```python
from build123d import *

# Parameters (mm, degrees)
F0_W     = 105.6
F0_H     = 55
F0_R     = 1.6
F0_R_2   = 21
F0_R_3   = 12.5
F1_DEPTH = 7
F2_R     = 3.1
F2_R_2   = 1.6
F3_DEPTH = 1.5
F4_W     = 6
F4_H     = 2.5
F5_DEPTH = 7.001
F7_DEPTH = 4
F8_R     = 1.75
F9_DEPTH = 55.001


with BuildPart() as f1:
    # F0 (on Top) → F1 (new body)
    with BuildSketch(Plane.XY):
        with Locations((50.8, 26.65)):
            Rectangle(F0_W, F0_H)
        with Locations((14, 2.5)):
            Circle(F0_R, mode=Mode.SUBTRACT)
        with Locations((66.1, 7.6)):
            Circle(F0_R, mode=Mode.SUBTRACT)
        with Locations((96.52, 2.5)):
            Circle(F0_R, mode=Mode.SUBTRACT)
        with Locations((40, 26.65)):
            Circle(F0_R_2, mode=Mode.SUBTRACT)
        with Locations((15.3, 50.7)):
            Circle(F0_R, mode=Mode.SUBTRACT)
        with Locations((66.1, 35.5)):
            Circle(F0_R, mode=Mode.SUBTRACT)
        with Locations((85, 26.65)):
            Circle(F0_R_3, mode=Mode.SUBTRACT)
        with Locations((90.2, 50.7)):
            Circle(F0_R, mode=Mode.SUBTRACT)
    extrude(amount=F1_DEPTH)

    # F2 (on face) → F3 (join)
    with BuildSketch(Plane.XY.offset(7)):
        with Locations((15.3, 50.7)):
            Circle(F2_R)
        with Locations((15.3, 50.7)):
            Circle(F2_R_2, mode=Mode.SUBTRACT)
        with Locations((90.2, 50.7)):
            Circle(F2_R)
        with Locations((90.2, 50.7)):
            Circle(F2_R_2, mode=Mode.SUBTRACT)
        with Locations((66.1, 35.5)):
            Circle(F2_R)
        with Locations((66.1, 35.5)):
            Circle(F2_R_2, mode=Mode.SUBTRACT)
        with Locations((66.1, 7.6)):
            Circle(F2_R)
        with Locations((66.1, 7.6)):
            Circle(F2_R_2, mode=Mode.SUBTRACT)
        with Locations((96.52, 2.5)):
            Circle(F2_R)
        with Locations((96.52, 2.5)):
            Circle(F2_R_2, mode=Mode.SUBTRACT)
        with Locations((14, 2.5)):
            Circle(F2_R)
        with Locations((14, 2.5)):
            Circle(F2_R_2, mode=Mode.SUBTRACT)
    extrude(amount=F3_DEPTH)

    # F4 (on face) → F5 (cut, through all)
    with BuildSketch(Plane.XY.offset(7)):
        with Locations((75.8, 48.9)):
            Rectangle(F4_W, F4_H)
        with Locations((75.8, 4.4)):
            Rectangle(F4_W, F4_H)
        with Locations((25.8, 48.9)):
            Rectangle(F4_W, F4_H)
        with Locations((25.8, 4.4)):
            Rectangle(F4_W, F4_H)
    extrude(amount=-F5_DEPTH, mode=Mode.SUBTRACT)

    # F6 (on face) → F7 (cut)
    with BuildSketch(Plane(origin=(0, 0, 0), x_dir=(1, 0, 0), z_dir=(0, 0, -1))):
        Polygon((12.267949, -5.5), (15.732051, -5.5), (17.464102, -2.5), (15.732051, 0.5), (12.267949, 0.5), (10.535898, -2.5), align=None)
        Polygon((98.252051, 0.5), (94.787949, 0.5), (93.055898, -2.5), (94.787949, -5.5), (98.252051, -5.5), (99.984102, -2.5), align=None)
        Polygon((63.1, -5.867949), (63.1, -9.332051), (66.1, -11.064102), (69.1, -9.332051), (69.1, -5.867949), (66.1, -4.135898), align=None)
        Polygon((63.1, -33.767949), (63.1, -37.232051), (66.1, -38.964102), (69.1, -37.232051), (69.1, -33.767949), (66.1, -32.035898), align=None)
        Polygon((91.932051, -47.7), (88.467949, -47.7), (86.735898, -50.7), (88.467949, -53.7), (91.932051, -53.7), (93.664102, -50.7), align=None)
        Polygon((13.567949, -47.7), (11.835898, -50.7), (13.567949, -53.7), (17.032051, -53.7), (18.764102, -50.7), (17.032051, -47.7), align=None)
    extrude(amount=-F7_DEPTH, mode=Mode.SUBTRACT)

    # F8 (on face) → F9 (cut, through all)
    with BuildSketch(Plane(origin=(0, 54.15, 0), x_dir=(-1, 0, 0), z_dir=(0, 1, 0))):
        with Locations((-75.8, 3.5)):
            Circle(F8_R)
        with Locations((-25.8, 3.5)):
            Circle(F8_R)
    extrude(amount=-F9_DEPTH, mode=Mode.SUBTRACT)


solid = f1.part
```
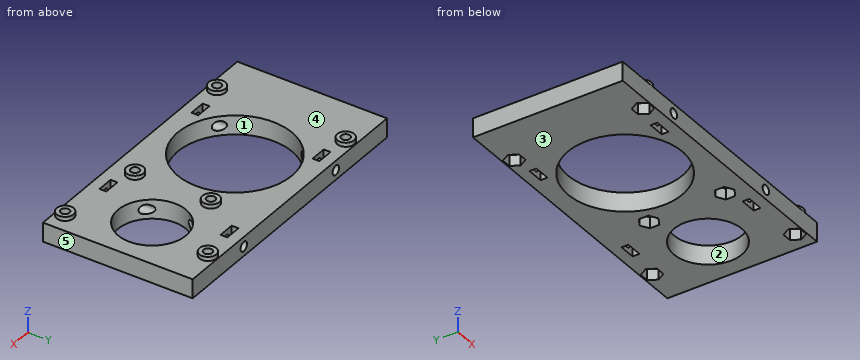
Could you check a few things on this model? Use its own coordinates, in mm. Face numbers are marked on the shaded views. A direction names the side the tool comes from. Round coordinates to 2 decimals unless told otherwise and drop trailing zeros. Order: outer loops, then holes, each group sorted by start corner. A loop starts at its lowest first (then second) coordinate and runs counter-clockwise, first axis right, second up. Notation, with made-up numbers: M -33,29.25 L 9,29.25 A17 ccw 9,52.25 Z; hole C -31.5,-36.75 d6. An arc over 180 degrees is marked long. One line per question, with ' | ' between items. Start each with the question number.
(1) Suppose I cut it at D-D on x = 90.2. List the corners of the cut face in (y, z) for me, then the cut area to 3 significant figures.
(2) Thinking about a two-plate mould opening in Y: for the marked faces 1, 2 and 3, which applies, +Y half, -Y half, draft (parallel to the pull), parting line (faces both ways), or undercut?
(3) Suppose I cut it at B-B on x = 40. List the corners of the cut face in (y, z) for me.
(4) Suppose I cut it at C-C on y = 7.6. List the corners of the cut face in (x, z) for me.
(5) Please list where these lines run through material, in increasing order: line 1 along X through (y, z) = (2.5, 6.7); line 2 along X through (y, z) = (50.7, 6.6); line 3 along Y through (x, z) = (40, 4.25).
(6) For P1, Ø5, axis at x = 76.5, z = 3, coming from the -Y side; P2, Ø4, axis at x = 44, y = 47.5, coming from the +Z side; P3, Ø1.9, axis at x = 90.2, y = 50.7, coming from the -Z side; P4, Ø5, axis at x = 15.3, y = 50.7, coming from the -Z side, each with a flat end and sliding along its axis, tell me the tip position at first contact or that it passes through.
(7) For the marked faces 4 and 5, which set-ups out of +Z, -Z, +X, -X, +Y, -Y let a thin tool reach every point of the face, with its end or its side?
(8) Suppose I cut it at A-A on y = 26.65. List the corners of the cut face in (x, z) for me, then the cut area to 3 significant figures.
Geometry results:
1) outline: M -0.85,0 L 15.28,0 L 15.28,7 L -0.85,7 Z; M 38.02,0 L 47.7,0 L 47.7,4 L 49.1,4 L 49.1,8.5 L 47.6,8.5 L 47.6,7 L 38.02,7 Z; M 52.3,4 L 53.7,4 L 53.7,0 L 54.15,0 L 54.15,7 L 53.8,7 L 53.8,8.5 L 52.3,8.5 Z | area: 197 mm²
2) face 1: undercut | face 2: undercut | face 3: draft
3) outline: M -0.85,0 L 5.65,0 L 5.65,7 L -0.85,7 Z; M 47.65,0 L 54.15,0 L 54.15,7 L 47.65,7 Z
4) outline: M -2,0 L 31.16,0 L 31.16,7 L -2,7 Z; M 48.84,0 L 63.1,0 L 63.1,4 L 64.5,4 L 64.5,8.5 L 63,8.5 L 63,7 L 48.84,7 Z; M 67.7,4 L 69.1,4 L 69.1,0 L 103.6,0 L 103.6,7 L 69.2,7 L 69.2,8.5 L 67.7,8.5 Z; hole C 25.8,3.5 d3.5; hole C 75.8,3.5 d3.5
5) line 1: -2 to 12.4, 15.6 to 94.92, 98.12 to 103.6 | line 2: -2 to 13.7, 16.9 to 88.6, 91.8 to 103.6 | line 3: -0.85 to 5.65, 47.65 to 54.15
6) P1: y = -0.85 | P2: z = 7 | P3: through | P4: z = 4
7) face 4: +Z | face 5: +Z, -Z, +X, +Y, -Y
8) outline: M -2,0 L 19,0 L 19,7 L -2,7 Z; M 61,0 L 72.5,0 L 72.5,7 L 61,7 Z; M 97.5,0 L 103.6,0 L 103.6,7 L 97.5,7 Z | area: 270 mm²
